The listing builds one solid part. Answer for the finished solid, in the listing's coordinates (mm). Round coordinates to 2 decimals unless told otherwise and drop trailing zeros. Loops run counter-clockwise (first coordinate to the right, second up) from the corner with the lowest first, then second, coordinate; pieces in that order, holes last. Notation, with made-up numbers: (-30, 61) - (24, 61) arc R21 ccw to (24, 91) - close; hole circle Ø9 at (63, 84.25). An arc over 180 degrees is marked (long way). Write item = value, one per line. Start each with the question number.
1) Section B-B, the plane x = 15 is taken. Determine the outline of the cut face in (y, z).
2) Straight lines are drawn through the part: line 1 along X through (y, z) = (2.45, 10.25); line 2 along X through (y, z) = (2.6, -1.5); line 3 along Z through (x, y) = (-16, 2.6). For each, find the intervals that lie inside material, in ascending order.
3) Section A-A, the plane y = 2.45 is taken. Determine the outline of the cut face in (x, z).
4) Given pin 1 Ø1.3 at (x, y) = (56, 3) entering from +Z; pin 2 Ø3 at (x, y) = (6, 4) entering from -Z; pin 3 Ø2.5 at (x, y) = (-38.5, 2) entering from -Z, each flat-ended and moving along its own axis, determine where each tip first touches the part or whether it passes through.
5) Section C-C, the plane x = -3 is taken. Determine the outline of the cut face in (y, z).
from build123d import *

# Parameters (mm, degrees)
ESQUISSE1_W        = 116
ESQUISSE1_H        = 5
BOSS_EXTRU_1_DEPTH = 10
ESQUISSE3_R        = 7.5
BOSS_EXTRU_3_DEPTH = 5


with BuildPart() as part:
    # Esquisse1 → Boss.-Extru.1 (new body)
    with BuildSketch(Plane.XY):
        with Locations((0, 2.5)):
            Rectangle(ESQUISSE1_W, ESQUISSE1_H)
    extrude(amount=BOSS_EXTRU_1_DEPTH)

    # Esquisse3 → Boss.-Extru.3 (add)
    with BuildSketch(Plane(origin=(0, 0, 0), x_dir=(1, 0, 0), z_dir=(0, 1, 0))):
        with Locations((-48, -5)):
            Circle(ESQUISSE3_R)
        with Locations((-24, -5)):
            Circle(ESQUISSE3_R)
        with Locations((0, -5)):
            Circle(ESQUISSE3_R)
        with Locations((24, -5)):
            Circle(ESQUISSE3_R)
        with Locations((48, -5)):
            Circle(ESQUISSE3_R)
    extrude(amount=BOSS_EXTRU_3_DEPTH)


solid = part.part
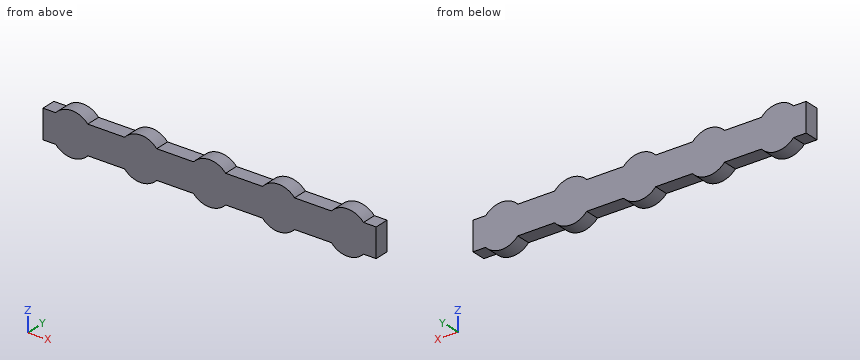
Geometry check:
q1.outline = (0, 0) - (5, 0) - (5, 10) - (0, 10) - close
q2.line_1 = -53.36 to -42.64, -29.36 to -18.64, -5.36 to 5.36, 18.64 to 29.36, 42.64 to 53.36
q2.line_2 = -51.74 to -44.26, -27.74 to -20.26, -3.74 to 3.74, 20.26 to 27.74, 44.26 to 51.74
q2.line_3 = 0 to 10
q3.outline = (-58, 0) - (-53.59, 0) arc R7.5 ccw to (-42.41, 0) - (-29.59, 0) arc R7.5 ccw to (-18.41, 0) - (-5.59, 0) arc R7.5 ccw to (5.59, 0) - (18.41, 0) arc R7.5 ccw to (29.59, 0) - (42.41, 0) arc R7.5 ccw to (53.59, 0) - (58, 0) - (58, 10) - (53.59, 10) arc R7.5 ccw to (42.41, 10) - (29.59, 10) arc R7.5 ccw to (18.41, 10) - (5.59, 10) arc R7.5 ccw to (-5.59, 10) - (-18.41, 10) arc R7.5 ccw to (-29.59, 10) - (-42.41, 10) arc R7.5 ccw to (-53.59, 10) - (-58, 10) - close
q4.pin_1 = 10
q4.pin_2 = -1
q4.pin_3 = 0
q5.outline = (0, -1.87) - (5, -1.87) - (5, 11.87) - (0, 11.87) - close
